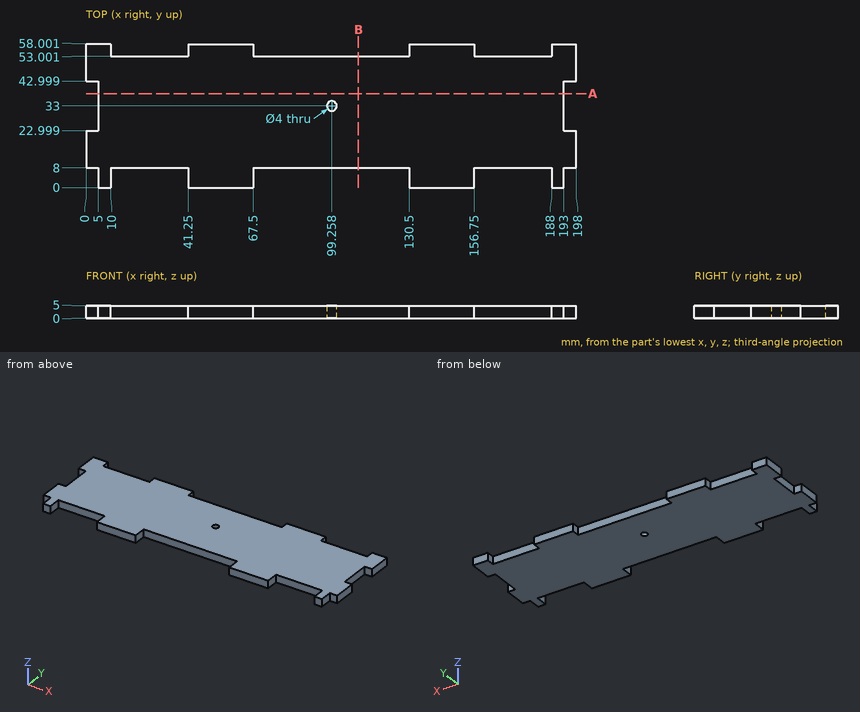
Part print with two shaded views. Sizes in mm from the minimum x, y, z corner. Coordinates: 2 decimals unless noted, no trailing zeros. Order: outer loops, then holes, each group sorted by start corner. A loop starts at its lowest first (then second) coordinate and runs counter-clockwise, first axis right, second up. Notation, with made-up numbers: (24, 63.25) - (53, 63.25) arc R19 ccw to (53, 74.25) - close; hole circle Ø10 at (-33.75, 58.5). An arc over 180 degrees is marked (long way). Answer in a Markdown table with one row per item.
1. Drill centre lines: L1, parallel to X at y = 54, z = 2.2; L2, parallel to X at y = 3, z = 3.8; L3, parallel to X at y = 24, z = 0.85. Where is each one in solid material? Low to high. Write a range as from..to.
Answer:
| item | result |
|---|---|
| L1 | 0..10, 41.25..67.5, 130.5..156.75, 188..198 |
| L2 | 5..10, 41.25..67.5, 130.5..156.75, 188..193 |
| L3 | 5..193 |
2. Slice it at B-B, the plane x = 110. List the corners of the cut face in (y, z), then the cut area to 3 significant figures.
Answer:
| item | result |
|---|---|
| outline | (8, 0) - (53, 0) - (53, 5) - (8, 5) - close |
| area | 225 mm² |
3. Flat gauge pins, fed straight in: P1, Ø2.5, axis at y = 54.5, z = 2.5, coming from the -X side; P2, Ø2.5, axis at y = 5, z = 2, coming from the -X side; P3, Ø1, axis at y = 35, z = 1.5, coming from the +X side. Where does each tip first touch, or does it go through?
Answer:
| item | result |
|---|---|
| P1 | x = 0 |
| P2 | x = 5 |
| P3 | x = 193 |
4. Slice it at A-A, the plane y = 38. List the corners of the cut face in (x, z).
Answer:
| item | result |
|---|---|
| outline | (5, 0) - (193, 0) - (193, 5) - (5, 5) - close |
